from build123d import *

# Parameters (mm, degrees)
SKETCH2_R           = 5.525
BOSS_EXTRUDE1_DEPTH = 10
SKETCH4_R           = 5.125
CUT_EXTRUDE2_DEPTH  = 7
SKETCH5_R           = 5.525
SKETCH5_R_2         = 4.5
BOSS_EXTRUDE4_DEPTH = 6


with BuildPart() as part:
    # Sketch2 → Boss-Extrude1 (new body)
    with BuildSketch(Plane.XY):
        with BuildLine():
            Line((-88.62562975, 0.527091372), (-88.62562975, -17.425503603))
            Line((-88.62562975, -17.425503603), (11.37437025, -17.425503603))
            Line((11.37437025, -17.425503603), (11.37437025, 2.574496397))
            Line((11.37437025, 2.574496397), (11.37437025, 66.938471641))
            ThreePointArc((11.37437025, 66.938471641), (2.08841102, 80.807492446), (-14.272261494, 77.504891684))
            Line((-14.272261494, 77.504891684), (-87.174506998, 4.049231386))
            ThreePointArc((-87.174506998, 4.049231386), (-88.248636685, 2.431771629), (-88.62562975, 0.527091372))
        make_face()
        with BuildLine():
            ThreePointArc((-55.776519908, 2.574496397), (-61.255836785, 6.063207717), (-60.051592087, 12.446295905))
            Line((-60.051592087, 12.446295905), (-15.620909093, 57.214260654))
            ThreePointArc((-15.620909093, 57.214260654), (-12.624755601, 58.661476378), (-9.38382576, 57.907989239))
            ThreePointArc((-9.38382576, 57.907989239), (-7.11800033, 56.813760216), (-4.659411057, 56.278371739))
            ThreePointArc((-4.659411057, 56.278371739), (-1.43979486, 54.662291481), (-0.142030474, 51.301718396))
            Line((-0.142030474, 51.301718396), (-0.142030474, 7.574496397))
            ThreePointArc((-0.142030474, 7.574496397), (-1.606496568, 4.038962491), (-5.142030474, 2.574496397))
            Line((-5.142030474, 2.574496397), (-55.776519908, 2.574496397))
        make_face(mode=Mode.SUBTRACT)
        with Locations((-3.62562975, 66.938471641)):
            Circle(SKETCH2_R, mode=Mode.SUBTRACT)
    extrude(amount=BOSS_EXTRUDE1_DEPTH)

    # Sketch4 → Cut-Extrude2 (cut)
    with BuildSketch(Plane.XZ.offset(17.425503603)):
        with Locations((-78.62562975, 2.5)):
            Circle(SKETCH4_R)
        with Locations((1.37437025, 2.5)):
            Circle(SKETCH4_R)
    extrude(amount=-CUT_EXTRUDE2_DEPTH, mode=Mode.SUBTRACT)

    # Sketch5 → Boss-Extrude4 (add)
    with BuildSketch(Plane(origin=(0, 0, 0), x_dir=(-1, 0, 0), z_dir=(0, 0, -1))):
        with Locations((3.62562975, 66.938471641)):
            Circle(SKETCH5_R)
        with Locations((3.62562975, 66.938471641)):
            Circle(SKETCH5_R_2, mode=Mode.SUBTRACT)
    extrude(amount=-BOSS_EXTRUDE4_DEPTH)


solid = part.part
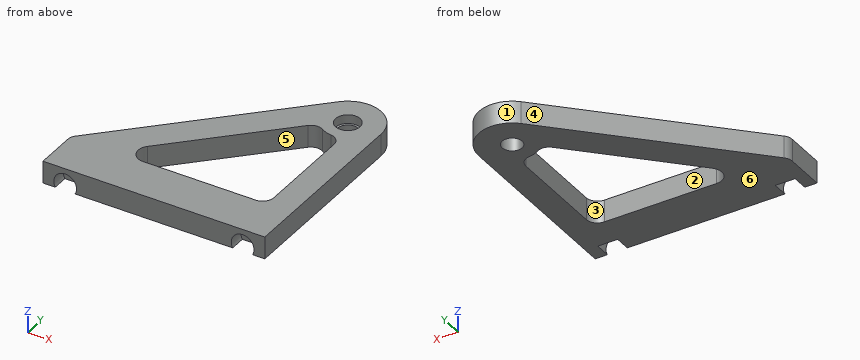
Here's how the part is built. I have some questions about the finished solid (model axes, mm). Face numbers are marked on the shaded views. A direction names the side the tool comes from. Give positions to 0.01 mm unless a question says otherwise; leave off trailing zeros. Order: outer loops, then holes, each group sorted by start corner. A loop starts at its lowest first (then second) coordinate and runs counter-clockwise, first axis right, second up. Notation, with made-up numbers: (58, 0.5) -> (101, 0.5) arc R26 cw to (101, 32.5) -> close; hole circle Ø11 at (83.25, 3.5). An arc over 180 degrees is marked (long way). Use a Markdown table: item, result. Add a question column.
Item 1: Will these pins go through, and if not, where does the flat tip stop? pin 1 (9 mm diameter, centred on x = -4, y = 66.5, fed in from +Z); pin 2 (3 mm diameter, centred on y = 37.5, z = 5, fed in from -X); pin 3 (6 mm diameter, centred on x = 2, z = 2, fed in from -Y).
Item 2: Imagine slicing it at B-B on y = 31.5. Please give me the cut outline in (x, z), plus the area to 3 significant figures.
Item 3: For the marked faces 1 and 2, which set-ups out of +Z, -Z, +X, -X, +Y, -Y let a thin tool reach every point of the face, with its end or its side?
Item 4: Imagine slicing it at D-D on y = 74.5. Please give me the cut outline in (x, z), plus the area to 3 significant figures.
Item 5: Imagine slicing it at A-A on z = 2.5. Please give me the cut outline in (x, y), plus the area to 3 significant figures.
Item 6: If we mould it in two halves opening along X, with no side actions, what happens to the marked faces 3, 4, 5 and 6? For each: pulls with the +X half, pulls with the -X half, needs draft (parallel to the pull), parting line crosses it, or undercut.
Item 7: Imagine slicing it at C-C on x = -12.5. Please give me the cut outline in (y, z), plus the area to 3 significant figures.
Item 8: I need wall thicknesses on line 1 (X direction, y = -15.25, z = 2.5); line 2 (X direction, y = -12, z = 2.75); line 3 (Y direction, x = -34, z = 6). Which ranges of each line are inside material? Lowest first, please.
Data:
| question | item | result |
|---|---|---|
| 1 | pin 1 | stops at z = 6 |
| 1 | pin 2 | stops at x = -55.46 |
| 1 | pin 3 | stops at y = -10.43 |
| 2 | outline | (-59.93, 0) -> (-41.14, 0) -> (-41.14, 10) -> (-59.93, 10) -> close; (-0.14, 0) -> (11.37, 0) -> (11.37, 10) -> (-0.14, 10) -> close |
| 2 | area | 303 mm² |
| 3 | face 1 | +Z, -Z, +Y |
| 3 | face 2 | +Z, -Z |
| 4 | outline | (-17.25, 0) -> (9.33, 0) -> (9.33, 10) -> (-17.25, 10) -> close |
| 4 | area | 266 mm² |
| 5 | outline | (-88.63, -17.43) -> (-83.75, -17.43) -> (-83.75, -10.43) -> (-73.5, -10.43) -> (-73.5, -17.43) -> (-3.75, -17.43) -> (-3.75, -10.43) -> (6.5, -10.43) -> (6.5, -17.43) -> (11.37, -17.43) -> (11.37, 66.94) arc R15 ccw to (-14.27, 77.5) -> (-87.17, 4.05) arc R5 ccw to (-88.63, 0.53) -> close; hole (-60.05, 12.45) arc R5.79 ccw to (-55.78, 2.57) -> (-5.14, 2.57) arc R5 ccw to (-0.14, 7.57) -> (-0.14, 51.3) arc R5 ccw to (-4.66, 56.28) arc R10.71 cw to (-9.38, 57.91) arc R5 ccw to (-15.62, 57.21) -> close; hole circle Ø9 at (-3.63, 66.94) |
| 5 | area | 4,270 mm² |
| 6 | face 3 | undercut |
| 6 | face 4 | pulls with the -X half |
| 6 | face 5 | undercut |
| 6 | face 6 | needs draft |
| 7 | outline | (-17.43, 0) -> (2.57, 0) -> (2.57, 10) -> (-17.43, 10) -> close; (58.67, 0) -> (79.03, 0) -> (79.03, 10) -> (58.67, 10) -> close |
| 7 | area | 404 mm² |
| 8 | line 1 | x = -88.63 to -83.75, -73.5 to -3.75, 6.5 to 11.37 |
| 8 | line 2 | x = -88.63 to -83.74, -73.51 to -3.74, 6.49 to 11.37 |
| 8 | line 3 | y = -17.43 to 2.57, 38.7 to 57.63 |
